Work out the finished part from the listing and answer in its coordinate system (mm). Face numbers are marked on the shaded views. A direction names the side the tool comes from. Round coordinates to 2 decimals unless told otherwise and drop trailing zeros. Write each loop counter-clockwise with the first axis right and the second up, starting at its lowest first coordinate (ties: lowest second). Pieces come first, ordered by that corner, then holes. Notation, with made-up numbers: M 29.25,63.25 L 42.25,63.25 A30 cw 42.25,91.25 Z; hole C -26.5,-4 d8. An arc over 180 degrees is marked long. Answer in a Markdown table with one row per item.
```python
from build123d import *

# Parameters (mm, degrees)
F0_R     = 11
F1_DEPTH = 1.5
F2_R     = 5
F3_DEPTH = 2.5
F4_R     = 2.6
F5_DEPTH = 4
F6_R     = 1


with BuildPart() as f1:
    # F0 (on Top) → F1 (new body)
    with BuildSketch(Plane.XY):
        Circle(F0_R)
    extrude(amount=-F1_DEPTH)

    # F2 (on face) → F3 (join)
    with BuildSketch(Plane.XY):
        Circle(F2_R)
    extrude(amount=F3_DEPTH)

    # F4 (on face) → F5 (cut)
    with BuildSketch(Plane.XY.offset(2.5)):
        Circle(F4_R)
    extrude(amount=-F5_DEPTH, mode=Mode.SUBTRACT)

    # F6
    f6_edges = [f1.edges().sort_by_distance(p)[0] for p in [
        (-11, 0, -1.5),
    ]]
    fillet(f6_edges, radius=F6_R)


solid = f1.part
```
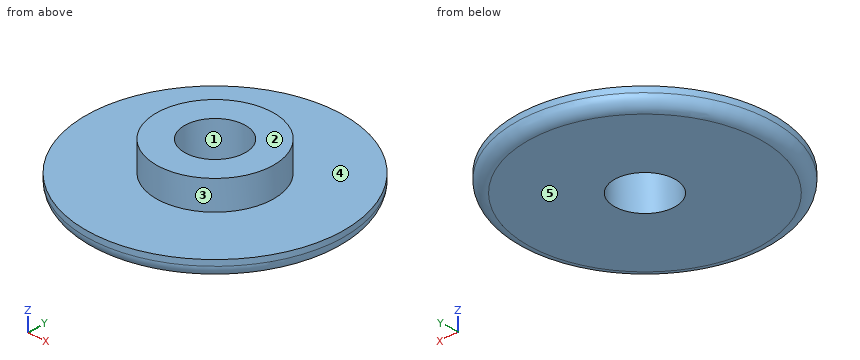
1. A tool of negligible diameter and unlimited length cuts with its end or side. For the marked faces 4 and 5, from which of +Z, -Z, +X, -X, +Y, -Y can it reach the whole face along a straight path? Write none if from no direction.
Calculated:
| item | result |
|---|---|
| face 4 | +Z |
| face 5 | -Z, +X, -X, +Y, -Y |
2. The part is cut by section A-A (x = 0). Determine the outline of the cut face in (y, z).
Calculated:
| item | result |
|---|---|
| outline | M -11,-0.5 A1 ccw -10,-1.5 L -2.6,-1.5 L -2.6,2.5 L -5,2.5 L -5,0 L -11,0 Z; M 2.6,-1.5 L 10,-1.5 A1 ccw 11,-0.5 L 11,0 L 5,0 L 5,2.5 L 2.6,2.5 Z |
3. Consider line 1 along Y through (x, z) = (0, 1.15); line 2 along Y through (x, z) = (-1.5, -0.65); line 3 along Z through (x, y) = (-2, 5). Determine where each line is inside the solid, lowest interval first. Write a range as from..to.
Calculated:
| item | result |
|---|---|
| line 1 | y = -5..-2.6, 2.6..5 |
| line 2 | y = -10.89..-2.12, 2.12..10.89 |
| line 3 | z = -1.5..0 |
4. Given pin 1 (1 mm diameter, centred on x = 4.5, z = 0, fed in from -Y); pin 2 (2 mm diameter, centred on y = 2, z = 1.5, fed in from -X), each flat-ended and moving along its own axis, determine where each tip first touches the part or whether it passes through.
Calculated:
| item | result |
|---|---|
| pin 1 | stops at y = -10.25 |
| pin 2 | stops at x = -4.9 |
5. Determine the mould class of the marked faces 1, 2 and 3 for opening direction X: released by +X, released by -X, zero draft, split by the parting line, or undercut.
Calculated:
| item | result |
|---|---|
| face 1 | undercut |
| face 2 | zero draft |
| face 3 | split by the parting line |
6. The part is cut by section C-C (z = 0.45). Determine the outline of the cut face in (x, y).
Calculated:
| item | result |
|---|---|
| outline | C 0,0 d10; hole C 0,0 d5.2 |
